Could you check a few things on this model? Use its own coordinates, in mm. Give positions to 0.01 mm unless a question says otherwise; leave off trailing zeros. Write each loop counter-clockwise with the first axis right and the second up, starting at its lowest first coordinate (ties: lowest second). Pieces come first, ordered by that corner, then holes. Notation, with made-up numbers: (50.5, 83.5) - (70.5, 83.5) arc R27 cw to (70.5, 122.5) - close; hole circle Ø11 at (48, 60). An arc over 180 degrees is marked (long way). Use one line per item in the form item = value.
```python
from build123d import *

# Parameters (mm, degrees)
SKETCH1_W           = 76
SKETCH1_H           = 55
BOSS_EXTRUDE1_DEPTH = 3
FILLET2_R           = 5
SKETCH2_R           = 3.175
CUT_EXTRUDE1_DEPTH  = 94.861600242


with BuildPart() as part:
    # Sketch1 → Boss-Extrude1 (new body)
    with BuildSketch(Plane(origin=(0, 0, 0), x_dir=(1, 0, 0), z_dir=(0, 1, 0))):
        with Locations((38, 27.5)):
            Rectangle(SKETCH1_W, SKETCH1_H)
    extrude(amount=BOSS_EXTRUDE1_DEPTH)

    # Fillet2
    fillet2_edges = [part.edges().sort_by_distance(p)[0] for p in [
        (0, 1.5, -55),
        (76, 1.5, -55),
        (76, 1.5, 0),
        (0, 1.5, 0),
    ]]
    fillet(fillet2_edges, radius=FILLET2_R)

    # Sketch2 → Cut-Extrude1 (cut, through all)
    with BuildSketch(Plane(origin=(0, 3, 0), x_dir=(1, 0, 0), z_dir=(0, 1, 0))):
        with Locations(Location((6.025, 48.1375, 0), (0, 0, 270))):
            Circle(SKETCH2_R)
        with Locations(Location((60, 48.1375, 0), (0, 0, 270))):
            Circle(SKETCH2_R)
        with Locations(Location((69.525, 48.1375, 0), (0, 0, 270))):
            Circle(SKETCH2_R)
        with Locations(Location((69.525, 6.8625, 0), (0, 0, 270))):
            Circle(SKETCH2_R)
        with Locations(Location((60, 6.8625, 0), (0, 0, 270))):
            Circle(SKETCH2_R)
        with Locations(Location((6.025, 6.8625, 0), (0, 0, 270))):
            Circle(SKETCH2_R)
    extrude(amount=-CUT_EXTRUDE1_DEPTH, mode=Mode.SUBTRACT)


solid = part.part
```
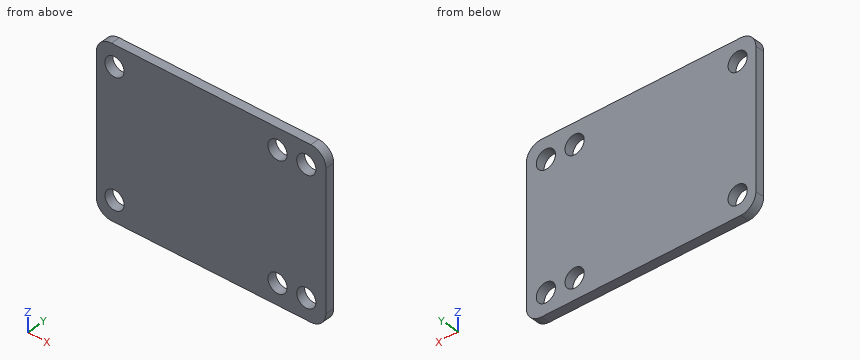
1. Imagine slicing it at D-D, the plane z = -47.5. List the corners of the cut face in (x, y) for me, and give its area (3 significant figures).
Response values:
outline = (0, 0) - (2.91, 0) - (2.91, 3) - (0, 3) - close; (9.14, 0) - (56.89, 0) - (56.89, 3) - (9.14, 3) - close; (63.11, 0) - (66.41, 0) - (66.41, 3) - (63.11, 3) - close; (72.64, 0) - (76, 0) - (76, 3) - (72.64, 3) - close
area = 172 mm²
2. If I drill on line 1 (X direction, y = 2.8, z = -48); line 2 (Z direction, x = 7, y = 1.6); line 3 (Z direction, x = 71, y = 1.15), over which ranges is the centre line in solid material (lowest first)? Write a range as from..to.
Response values:
line_1 = 0..2.85, 9.2..56.83, 63.17..66.35, 72.7..76
line_2 = -55..-51.16, -45.12..-9.88, -3.84..0
line_3 = -55..-50.95, -45.33..-9.67, -4.05..0
3. Imagine slicing it at B-B, the plane z = -9. List the corners of the cut face in (x, y) for me.
Response values:
outline = (0, 0) - (3.68, 0) - (3.68, 3) - (0, 3) - close; (8.37, 0) - (57.65, 0) - (57.65, 3) - (8.37, 3) - close; (62.35, 0) - (67.18, 0) - (67.18, 3) - (62.35, 3) - close; (71.87, 0) - (76, 0) - (76, 3) - (71.87, 3) - close
4. Imagine slicing it at A-A, the plane x = 60. List the corners of the cut face in (y, z) for me, and give its area (3 significant figures).
Response values:
outline = (0, -55) - (3, -55) - (3, -51.31) - (0, -51.31) - close; (0, -44.96) - (3, -44.96) - (3, -10.04) - (0, -10.04) - close; (0, -3.69) - (3, -3.69) - (3, 0) - (0, 0) - close
area = 127 mm²
5. Imagine slicing it at C-C, the plane y = 2.05. State how many separate pieces and enclosed holes the cut face has, and give its area (3 significant figures).
Response values:
separate_pieces = 1
enclosed_holes = 6
area = 3,970 mm²
6. For pin 1 (7.5 mm diameter, centred on x = 69.53, z = -48.14, fed in from -Y), with a flat end and sliding along its axis, tell me the tip position at first contact or that it passes through.
Response values:
pin_1 = 0
